from build123d import *

# Parameters (mm, degrees)
F0_W     = 203.2
F0_H     = 38.1
F1_DEPTH = 127
F2_R     = 15.875
F3_DEPTH = 127.001
F4_SIZE  = 3.048
F5_R     = 26.19375
F6_DEPTH = 38.101
F7_ANGLE = 90


with BuildPart() as f1:
    # F0 (on Top) → F1 (new body)
    with BuildSketch(Plane.XY):
        with Locations((-80.2247157872, -0.3943982914)):
            Rectangle(F0_W, F0_H)
    extrude(amount=F1_DEPTH)

    # F2 (on face) → F3 (cut, through all)
    with BuildSketch(Plane.XY.offset(127)):
        with Locations((-156.4247157872, -0.3943982914)):
            Circle(F2_R)
        with Locations((-4.0247157872, -0.3943982914)):
            Circle(F2_R)
    extrude(amount=-F3_DEPTH, mode=Mode.SUBTRACT)

    # F4
    f4_edges = [f1.edges().sort_by_distance(p)[0] for p in [
        (-181.824716, -19.444398, 63.5),
        (21.375284, -19.444398, 63.5),
        (21.375284, 18.655602, 63.5),
        (-181.824716, 18.655602, 63.5),
    ]]
    chamfer(f4_edges, length=F4_SIZE)

    # F5 (on face) → F6 (cut, through all)
    with BuildSketch(Plane.XZ.offset(19.4443982914)):
        with Locations((-80.2247157872, 38.1)):
            Circle(F5_R)
    extrude(amount=-F6_DEPTH, mode=Mode.SUBTRACT)


with BuildPart() as f1_1:
    # F7: moved
    add(f1.part.rotate(Axis((18.3272842128, -19.4443982914, 63.5), (0, 0, 1)), F7_ANGLE))


solid = f1_1.part
Geometry check sheet. Reference: the model listing, model coordinates, mm. Give positions to 0.01 mm unless a question says otherwise; leave off trailing zeros. Order: outer loops, then holes, each group sorted by start corner. A loop starts at its lowest first (then second) coordinate and runs counter-clockwise, first axis right, second up. Notation, with made-up numbers: M -11.75,29 L 32.25,29 A16 cw 32.25,41 Z; hole C 60.5,74 d9. An arc over 180 degrees is marked long. Use a Markdown table: item, result.
Item 1: Section check B-B (z = 26). Record the cut outline in (x, y) (3 decimals).
Answers follow:
| item | result |
|---|---|
| outline | M -19.773,-216.548 L -16.725,-219.596 L 15.279,-219.596 L 18.327,-216.548 L 18.327,-141.228 L -19.773,-141.228 Z; M -19.773,-94.765 L 18.327,-94.765 L 18.327,-19.444 L 15.279,-16.396 L -16.725,-16.396 L -19.773,-19.444 Z; hole C -0.723,-194.196 d31.75; hole C -0.723,-41.796 d31.75 |
Item 2: Material ranges on line 1 along Y through (x, z) = (6.5, 91); line 2 along Y through (x, z) = (-9.5, 105); line 3 along Y through (x, z) = (-1, 43), recorded low to high.
Answers follow:
| item | result |
|---|---|
| line 1 | y = -219.6 to -208.33, -180.06 to -55.93, -27.66 to -16.4 |
| line 2 | y = -219.6 to -207.42, -180.97 to -55.02, -28.57 to -16.4 |
| line 3 | y = -219.6 to -210.07, -178.32 to -143.73, -92.27 to -57.67, -25.92 to -16.4 |
Item 3: Section check C-C (x = -12). Record the cut outline in (y, z), and give its area (3 significant figures).
Answers follow:
| item | result |
|---|---|
| outline | M -219.6,0 L -205.37,0 L -205.37,127 L -219.6,127 Z; M -183.02,0 L -52.97,0 L -52.97,127 L -183.02,127 Z; M -30.62,0 L -16.4,0 L -16.4,127 L -30.62,127 Z; hole C -118,38.1 d52.39 |
| area | 18,000 mm2 |
Item 4: Section check D-D (z = 108). Record the cut outline in (x, y) (3 decimals).
Answers follow:
| item | result |
|---|---|
| outline | M -19.773,-216.548 L -16.725,-219.596 L 15.279,-219.596 L 18.327,-216.548 L 18.327,-19.444 L 15.279,-16.396 L -16.725,-16.396 L -19.773,-19.444 Z; hole C -0.723,-194.196 d31.75; hole C -0.723,-41.796 d31.75 |
Item 5: Section check A-A (y = -118). Record the cut outline in (x, z), and give its area (3 significant figures).
Answers follow:
| item | result |
|---|---|
| outline | M -19.77,0 L 18.33,0 L 18.33,11.91 L -19.77,11.91 Z; M -19.77,64.29 L 18.33,64.29 L 18.33,127 L -19.77,127 Z |
| area | 2,840 mm2 |
Item 6: Draft check along X on faces 1 (the cylindrical face through (-1.421, -57.656, 64.389)), 2 (the flat face through (-19.773, -119, 77)), 3 (the flat face through (-1, -119, 0)), 4 (the cylindrical face through (-5.491, -179.054, 64.389)). Enter one of: +X half, -X half, draft (parallel to the pull), parting line (faces both ways), or undercut.
Answers follow:
| item | result |
|---|---|
| face 1 | undercut |
| face 2 | -X half |
| face 3 | draft |
| face 4 | undercut |
Item 7: Depth check by flat-ended pin: P1, Ø19, axis at x = -0.72, y = -41.8, coming from the -Z side. Enter the tip coordinate at first touch or a pass-through.
Answers follow:
| item | result |
|---|---|
| P1 | passes through |
